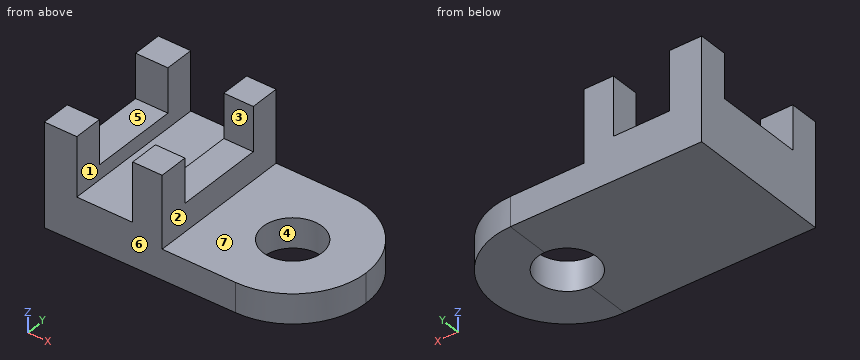
```python
from build123d import *

# Parameters (mm, degrees)
F1_DEPTH = 63.5
F3_DEPTH = 12.7
F4_R     = 12.7
F6_DEPTH = 25.4
F5_W     = 38.1
F5_H     = 19.05
F7_DEPTH = 50.801


with BuildPart() as f1:
    # F0 (on Front) → F1 (new body)
    with BuildSketch(Plane.XZ):
        Polygon((5.667796, 17.475092), (-8.302204, 17.475092), (-8.302204, -26.974908), (74.245038, -26.300137), (74.245038, -13.600137), (42.497796, -13.600137), (42.497796, 17.475092), (29.797796, 17.475092), (29.797796, -7.924908), (5.667796, -7.924908), align=None)
    extrude(amount=F1_DEPTH)

    # F2 (on face) → F3 (join)
    with BuildSketch(Plane.XY.offset(-13.600137)):
        with BuildLine():
            ThreePointArc((74.245038, -63.5), (96.695679, -54.20064), (105.995038, -31.75))
            ThreePointArc((105.995038, -31.75), (96.695679, -9.29936), (74.245038, 0))
            Line((74.245038, 0), (74.245038, -63.5))
        make_face()
    extrude(amount=-F3_DEPTH)

    # F4 (on face) → F6 (cut)
    with BuildSketch(Plane.XY.offset(-13.600137)):
        with Locations((74.245038, -31.75)):
            Circle(F4_R)
    extrude(amount=-F6_DEPTH, mode=Mode.SUBTRACT)

    # F5 (on face) → F7 (cut, through all)
    with BuildSketch(Plane.YZ.offset(42.497796)):
        with Locations((-31.75, 7.950092)):
            Rectangle(F5_W, F5_H)
    extrude(amount=-F7_DEPTH, mode=Mode.SUBTRACT)


solid = f1.part
```
CAD build for the part. Positions are in the model's coordinates, mm. Face numbers are marked on the shaded views. A direction names the side the tool comes from. Give positions to 0.01 mm unless a question says otherwise; leave off trailing zeros. Order: outer loops, then holes, each group sorted by start corner. A loop starts at its lowest first (then second) coordinate and runs counter-clockwise, first axis right, second up. Notation, with made-up numbers: M -11,83.5 L 22,83.5 A3 ccw 22,87.5 Z; hole C 19,21 d7. An arc over 180 degrees is marked long. Put each result on its own line as item: value. Start each with the question number.
(1) Saw through at B-B, the plane y = -34.5. Write the cut outline in (x, z).
(2) Saw through at A-A, the plane z = 11. Write the cut outline in (x, y), then the cut area to 3 significant figures.
(3) Saw through at D-D, the plane y = -20.5. Write the cut outline in (x, z), then the cut area to 3 significant figures.
(4) Drill centre lines: line 1 along X through (y, z) = (-60, -7); line 2 along X through (y, z) = (-31.75, -23.5); line 3 along Y through (x, z) = (40, 8). Where is each one in solid material? Low to high.
(5) Mould opens along Y. For the marked faces 4, 5, 6 and 7 say: +Y half, -Y half, draft (parallel to the pull), parting line (faces both ways), or undercut.
(6) Which spindle directions (+Z, -Z, +X, -X, +Y, -Y) get a long thin tool onto all of the face, cutting with end or side? Do the marked faces 1, 2 and 3. Say none if no direction does.
(7) Saw through at C-C, the plane z = -23. Write the cut outline in (x, y), then the cut area to 3 significant figures.
(8) Flat gauge pins, fed straight in: pin 1 Ø11 at (x, z) = (-3, 7.5) entering from +Y; pin 2 Ø6 at (x, y) = (17.5, -53) entering from +Z; pin 3 Ø20.5 at (y, z) = (-25, 5) entering from +X; pin 4 Ø9.5 at (y, z) = (-21, 7.5) entering from +X. Where does each tip first touch, or does it go through?
Check result:
1. outline: M -8.3,-26.97 L 61.85,-26.4 L 61.85,-13.6 L 42.5,-13.6 L 42.5,-1.57 L 29.8,-1.57 L 29.8,-7.92 L 5.67,-7.92 L 5.67,-1.57 L -8.3,-1.57 Z; M 86.64,-26.3 L 105.88,-26.3 L 105.88,-13.6 L 86.64,-13.6 Z
2. outline: M -8.3,-63.5 L 5.67,-63.5 L 5.67,-50.8 L -8.3,-50.8 Z; M -8.3,-12.7 L 5.67,-12.7 L 5.67,0 L -8.3,0 Z; M 29.8,-63.5 L 42.5,-63.5 L 42.5,-50.8 L 29.8,-50.8 Z; M 29.8,-12.7 L 42.5,-12.7 L 42.5,0 L 29.8,0 Z
2. area: 677 mm2
3. outline: M -8.3,-26.97 L 68.35,-26.35 L 68.35,-13.6 L 42.5,-13.6 L 42.5,-1.57 L 29.8,-1.57 L 29.8,-7.92 L 5.67,-7.92 L 5.67,-1.57 L -8.3,-1.57 Z; M 80.14,-26.3 L 103.94,-26.3 L 103.94,-13.6 L 80.14,-13.6 Z
3. area: 1,760 mm2
4. line 1: x = -8.3 to 5.67, 29.8 to 42.5
4. line 2: x = -8.3 to 61.55, 86.95 to 106
4. line 3: y = -63.5 to -50.8, -12.7 to 0
5. face 4: undercut
5. face 5: undercut
5. face 6: -Y half
5. face 7: draft
6. face 1: +Z, +Y, -Y
6. face 2: +Z, +X, +Y, -Y
6. face 3: +Z, +X, -X
7. outline: M -8.3,-63.5 L 74.25,-63.5 A31.75 ccw 106,-31.75 A31.75 ccw 74.25,0 L -8.3,0 Z; hole C 74.25,-31.75 d25.4
7. area: 6,320 mm2
8. pin 1: stops at y = 0
8. pin 2: stops at z = -7.92
8. pin 3: stops at x = 42.5
8. pin 4: passes through
